Here's the drawing with two shaded views (mm, measured from the low corner). I have some questions. A direction names the side the tool comes from. Give positions to 0.01 mm unless a question says otherwise; leave off trailing zeros. Loops run counter-clockwise (first coordinate to the right, second up) from the corner with the lowest first, then second, coordinate; pieces in that order, holes last.
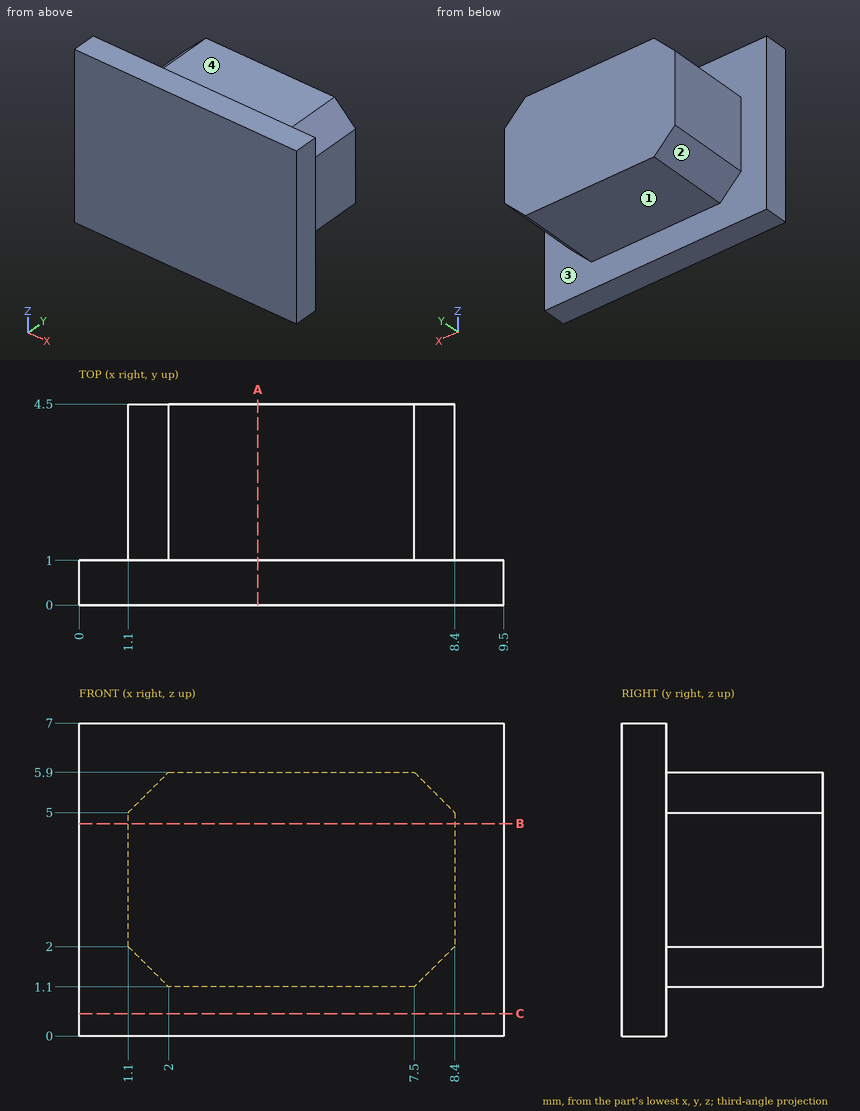
(1) Please list where these lines run through material, in increasing order: probe 1 along X at (y, z) = (4.35, 4.25); probe 2 along Y at (x, z) = (8.25, 6); probe 3 along Z at (x, y) = (6.5, 1.15).
Returned:
probe 1: x = 1.1 to 8.4
probe 2: y = 0 to 1
probe 3: z = 1.1 to 5.9
(2) Which directions (+Z, -Z, +X, -X, +Y, -Y) give clear straight access to the entire face, cutting with the end or side of a thin tool? Please do the marked faces 1, 2, 3 and 4.
Returned:
face 1: -Z, +X, -X, +Y
face 2: -Z, -X, +Y
face 3: +Y
face 4: +Z, +X, -X, +Y
(3) Suppose I cut it at C-C on z = 0.5. List the corners of the cut face in (x, y) for me, plus the area to 3 significant figures.
Returned:
outline: (0, 0) - (9.5, 0) - (9.5, 1) - (0, 1) - close
area: 9.50 mm2
(4) Will these pins go through, and if not, where does the flat tip stop? P1, Ø1, axis at x = 5, y = 2.5, coming from the -Z side; P2, Ø1.5, axis at y = 3, z = 3.5, coming from the +X side.
Returned:
P1: stops at z = 1.1
P2: stops at x = 8.4
(5) Suppose I cut it at A-A on x = 4. List the corners of the cut face in (y, z) for me.
Returned:
outline: (0, 0) - (1, 0) - (1, 1.1) - (4.5, 1.1) - (4.5, 5.9) - (1, 5.9) - (1, 7) - (0, 7) - close
(6) Suppose I cut it at B-B on z = 4.75. List the corners of the cut face in (x, y) for me, plus the area to 4 significant figures.
Returned:
outline: (0, 0) - (9.5, 0) - (9.5, 1) - (8.4, 1) - (8.4, 4.5) - (1.1, 4.5) - (1.1, 1) - (0, 1) - close
area: 35.05 mm2
